The drawing under review shows one solid part. Ordinate dimensions are in mm from its lowest x, y, z. Give positions to 0.01 mm unless a question says otherwise; leave off trailing zeros. Write each loop counter-clockwise with the first axis right and the second up, starting at its lowest first coordinate (ties: lowest second). Pieces come first, ordered by that corner, then holes.
Q1. We need section B-B (x = 12.7). Write out the cut boundary in (y, z).
Q2. For line 1 (Y direction, x = 12.7, z = 9.5); line 2 (Y direction, x = 13.5, z = 23); line 3 (Y direction, x = 24.25, z = 5.5), list the stretches that pass through material, from the lowest coordinate up.
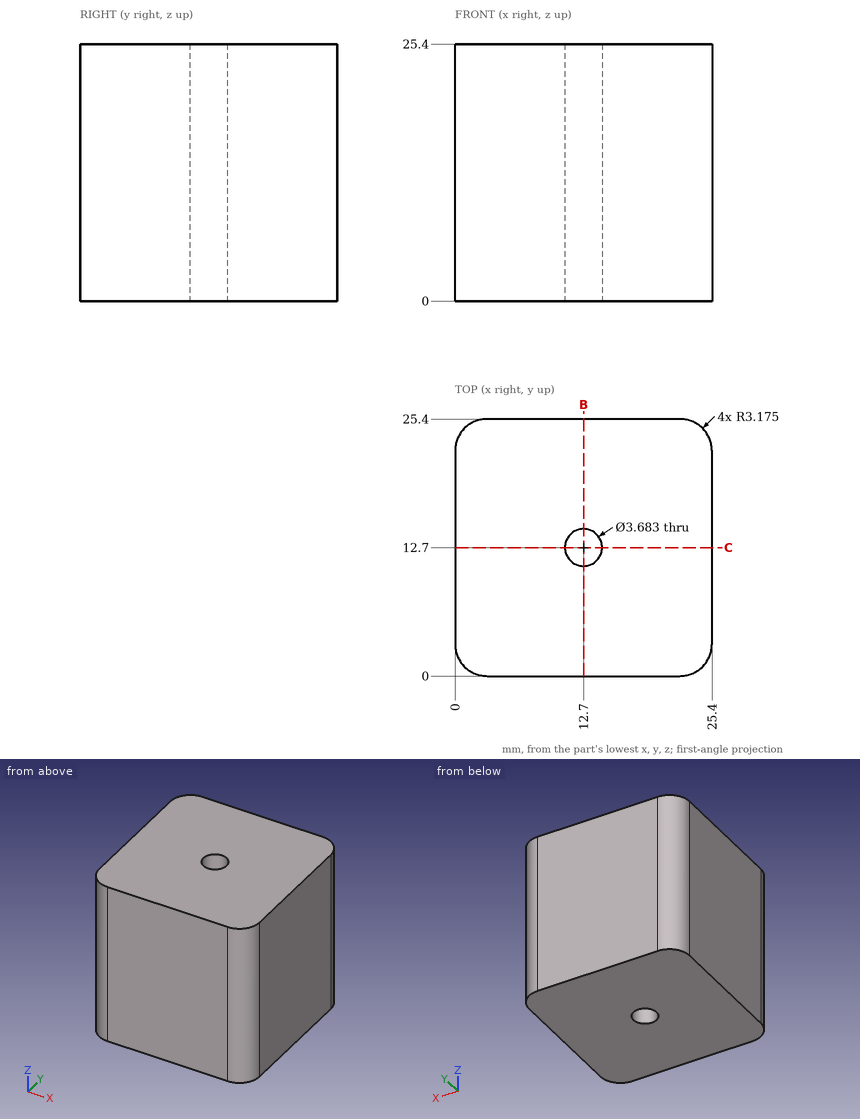
Computed:
1. outline: (0, 0) - (10.86, 0) - (10.86, 25.4) - (0, 25.4) - close; (14.54, 0) - (25.4, 0) - (25.4, 25.4) - (14.54, 25.4) - close
2. line 1: y = 0 to 10.86, 14.54 to 25.4
2. line 2: y = 0 to 11.04, 14.36 to 25.4
2. line 3: y = 0.73 to 24.67
